```python
from build123d import *

# Parameters (mm, degrees)
F0_R      = 41.275
F0_R_2    = 12.7
F1_DEPTH  = 19.05
F2_SIZE2  = 0.3402954744
F2_SIZE   = 1.27
F4_D      = 3.4544
F4_DEPTH  = 11.43
F4_TIP    = 1.0378064612
F6_D      = 3.4544
F6_DEPTH  = 15.24
F6_TIP    = 1.0378064612
F8_D      = 4.4958
F9_R      = 28.0416
F9_R_2    = 22.7076
F10_DEPTH = 2.6924
F11_R     = 0.7874


with BuildPart() as f1:
    # F0 (on Top) → F1 (new body)
    with BuildSketch(Plane.XY):
        Circle(F0_R)
        Circle(F0_R_2, mode=Mode.SUBTRACT)
    extrude(amount=F1_DEPTH)

    # F2
    f2_edges = [f1.edges().sort_by_distance(p)[0] for p in [
        (-12.7, 0, 19.05),
        (-12.7, 0, 0),
    ]]
    f2_side = f1.faces().sort_by_distance((-12.7, 0, 9.525))[0]
    chamfer(f2_edges, length=F2_SIZE, length2=F2_SIZE2, reference=f2_side)

    # F4
    with Locations(Plane(origin=(0, 0, 0), x_dir=(1, 0, 0), z_dir=(0, 0, -1))):
        with Locations((0, -17.78), (-17.78, 0), (0, 17.78), (17.78, 0)):
            Hole(F4_D / 2, depth=F4_DEPTH)
            with Locations((0, 0, -(F4_DEPTH + F4_TIP / 2))):  # 118° drill point
                Cone(0, F4_D / 2, F4_TIP, mode=Mode.SUBTRACT)

    # F6
    with Locations(Plane.XY.offset(19.05)):
        with Locations((35, 0), (0, -35), (-35, 0), (0, 35)):
            Hole(F6_D / 2, depth=F6_DEPTH)
            with Locations((0, 0, -(F6_DEPTH + F6_TIP / 2))):  # 118° drill point
                Cone(0, F6_D / 2, F6_TIP, mode=Mode.SUBTRACT)

    # F8 (through all)
    with Locations(Plane.XY.offset(19.05)):
        with Locations((24.7487373415, -24.7487373415), (-24.7487373415, -24.7487373415), (-24.7487373415, 24.7487373415), (24.7487373415, 24.7487373415)):
            Hole(F8_D / 2)

    # F9 (on face) → F10 (cut)
    with BuildSketch(Plane(origin=(0, 0, 0), x_dir=(1, 0, 0), z_dir=(0, 0, -1))):
        Circle(F9_R)
        Circle(F9_R_2, mode=Mode.SUBTRACT)
    extrude(amount=-F10_DEPTH, mode=Mode.SUBTRACT)

    # F11
    f11_edges = [f1.edges().sort_by_distance(p)[0] for p in [
        (-22.7076, 0, 2.6924),
        (-28.0416, 0, 2.6924),
    ]]
    fillet(f11_edges, radius=F11_R)


solid = f1.part
```
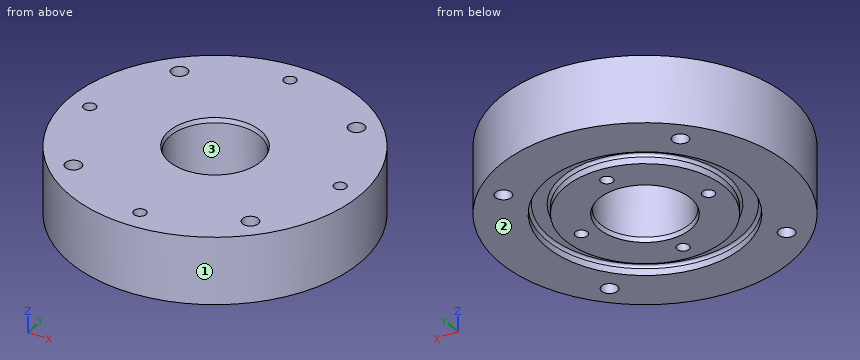
For this review, take the finished solid that the model builds, in its own axes (mm). Face numbers are marked on the shaded views. Round coordinates to 2 decimals unless told otherwise and drop trailing zeros. Write each loop counter-clockwise with the first axis right and the second up, starting at its lowest first coordinate (ties: lowest second). Pieces come first, ordered by that corner, then holes. Notation, with made-up numbers: (59, -4) -> (96, -4) arc R21 ccw to (96, 9) -> close; hole circle Ø7 at (60.5, 58). An arc over 180 degrees is marked (long way). Use one line per item in the form item = value.
Q1. Clearance check with flat-ended pins moving along their axes: pin 1 Ø5 at (y, z) = (-13.5, 13) entering from +X; pin 2 Ø23 at (x, y) = (0, 0) entering from +Z; pin 3 Ø8 at (x, z) = (30.5, 4) entering from +Y; pin 4 Ø5 at (y, z) = (11.5, 2) entering from +X. State where each tip first meets the part, or that it passes through.
Resolved:
pin_1 = 39.78
pin_2 = through
pin_3 = 31.64
pin_4 = 40.28
Q2. To check wall thickness, follow probe 1 along Y at (x, z) = (-1.5, 12.5); probe 2 along X at (y, z) = (-25, 15.75); probe 3 along X at (y, z) = (1, 9.75). State the ranges of each line that lie inside material, in increasing order. Write a range as from..to.
Resolved:
probe_1 = -41.25..-35.86, -34.14..-12.61, 12.61..34.14, 35.86..41.25
probe_2 = -32.84..-26.98, -22.51..22.51, 26.98..32.84
probe_3 = -41.26..-36.41, -33.59..-19.19, -16.37..-12.66, 12.66..16.37, 19.19..33.59, 36.41..41.26
Q3. Consider section C-C (y = 31.5). State the section outline as (x, z) points, then the cut area to 3 significant figures.
Resolved:
outline = (-26.67, 0) -> (26.67, 0) -> (26.67, 19.05) -> (-26.67, 19.05) -> close
area = 1,020 mm²
Q4. The part is to be moulded in two halves that separate along Y. For the marked faces 1, 2 and 3, say which applies: released by +Y, released by -Y, zero draft, split by the parting line, or undercut.
Resolved:
face_1 = split by the parting line
face_2 = zero draft
face_3 = undercut
Q5. Consider section A-A (z = 14.75). State how many separate pieces and enclosed holes the cut face has, then the cut area to 3 significant figures.
Resolved:
separate_pieces = 1
enclosed_holes = 9
area = 4,740 mm²
Q6. Consider section D-D (x = -31). State the section outline as (y, z) points, then the cut area to 3 significant figures.
Resolved:
outline = (-27.25, 0) -> (27.25, 0) -> (27.25, 19.05) -> (-27.25, 19.05) -> close
area = 1,040 mm²
